Drawing for the job (mm, zero at the part's lowest x, y, z). Round coordinates to 2 decimals unless told otherwise and drop trailing zeros. Order: outer loops, then holes, each group sorted by start corner. A loop starts at its lowest first (then second) coordinate and runs counter-clockwise, first axis right, second up. Notation, with made-up numbers: (60.25, 15.25) - (70.25, 15.25) arc R15 cw to (70.25, 27.25) - close; hole circle Ø3 at (60.25, 28). An arc over 180 degrees is marked (long way). One line per question, with ' | ' between items. Start each with the question number.
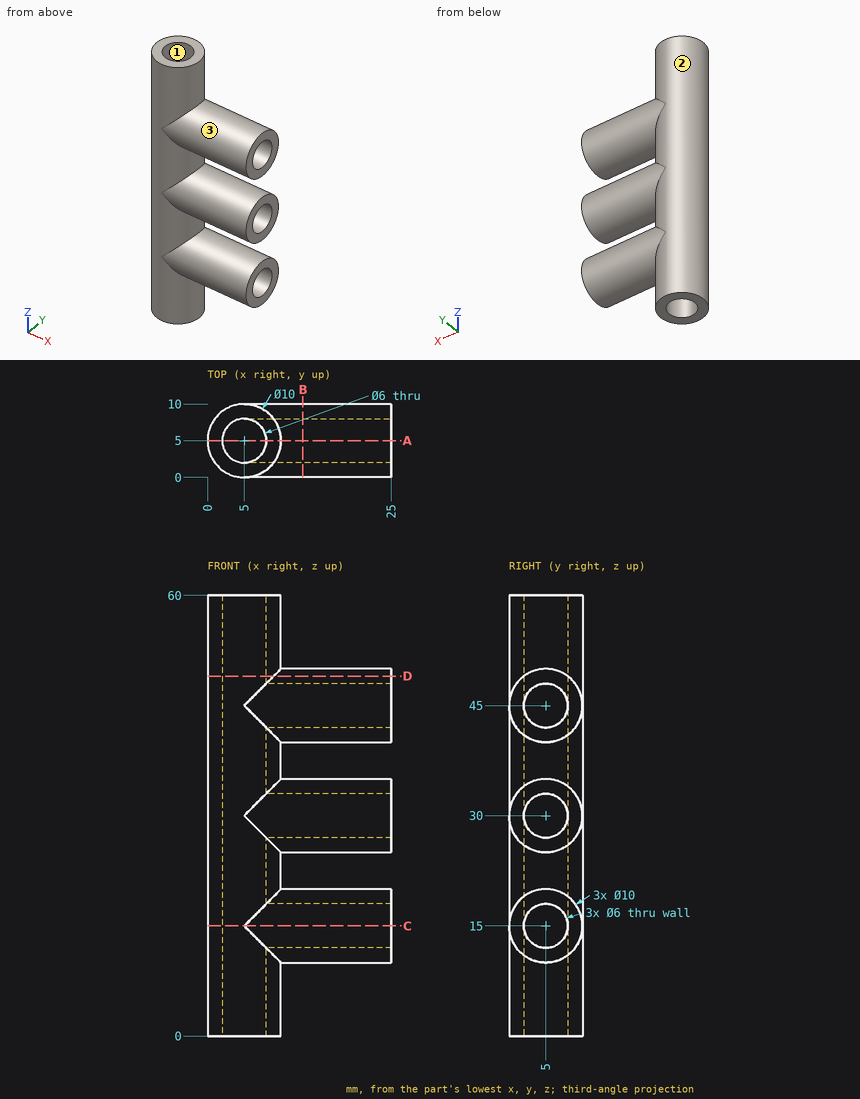
Item 1: Wall check: line 1 along Z through (x, y) = (12.25, 5); line 2 along Y through (x, z) = (5, 29); line 3 along Z through (x, y) = (8.5, 2.5). Give the ranges that are in metal, low to high. Write a range as [from, to].
Item 2: Slice it at D-D (z = 49). Write the cut outline in (x, y).
Item 3: Slice it at C-C (z = 15). Write the cut outline in (x, y), plus the area to 3 significant figures.
Item 4: Slice it at A-A (y = 5). Count the separate pieces of the cut face and the enclosed holes in it, plus the area to 3 significant figures.
Item 5: Slice it at B-B (x = 13). Write the cut outline in (y, z), plus the area to 3 significant figures.
Item 6: Pin check, flat tips, straight feed: pin 1 (1 mm diameter, centred on y = 3.5, z = 42.5, fed in from +X); pin 2 (3.5 mm diameter, centred on y = 5, z = 30, fed in from +X); pin 3 (1.5 mm diameter, centred on x = 20, z = 9, fed in from +Y); pin 4 (1.5 mm diameter, centred on x = 16.5, y = 2, fed in from +Z). Stop position of each tip, or through.
Item 7: Pull direction X, two halves, no side cores. Call the marked faces 1, 2 and 3: released by +X, released by -X, zero draft, split by the parting line, or undercut.
A:
1) line 1: [10, 12], [18, 20], [25, 27], [33, 35], [40, 42], [48, 50] | line 2: [0, 2], [8, 10] | line 3: [0, 13.34], [16.66, 28.34], [31.66, 43.34], [46.66, 60]
2) outline: (9, 2) - (25, 2) - (25, 8) - (9, 8) arc R5 ccw (long way) to start; hole circle Ø6 at (5, 5)
3) outline: (5, 0) - (25, 0) - (25, 2) - (5, 2) arc R3 cw to (5, 8) - (25, 8) - (25, 10) - (5, 10) arc R5 ccw to start | area: 105 mm^2
4) separate pieces: 5 | enclosed holes: 0 | area: 384 mm^2
5) outline: circle Ø10 at (5, 15); circle Ø10 at (5, 30); circle Ø10 at (5, 45); hole circle Ø6 at (5, 15); hole circle Ø6 at (5, 30); hole circle Ø6 at (5, 45) | area: 151 mm^2
6) pin 1: x = 25 | pin 2: x = 2.56 | pin 3: through | pin 4: z = 49.47
7) face 1: undercut | face 2: split by the parting line | face 3: zero draft
